from build123d import *

# Parameters (mm, degrees)
CORPS_D_PLACER_COPIER2_DEPTH = 104.8
BOSS_EXTRU_1_DEPTH           = 20
BOSS_EXTRU_1_DEPTH_BACK      = 130
ESQUISSE1_R                  = 5


with BuildPart() as part:
    # Corps-Déplacer/Copier2: read off the stored shape, not the designer's step
    # Corps-Déplacer/Copier2 outline → Corps-Déplacer/Copier2 (new body)
    with BuildSketch(Plane(origin=(0, 0, 0), x_dir=(1, 0, 0), z_dir=(0, 1, 0))):
        Polygon((7, 7), (-7, 7), (-7, -7), (7, -7), (11, 0), align=None)
    extrude(amount=CORPS_D_PLACER_COPIER2_DEPTH)

    # Corps-D_placer_Copier2 2 outline → Corps-D_placer_Copier2 2 (revolve, cut)
    with BuildSketch(Plane.XY):
        with BuildLine():
            Line((11, 104.8), (5, 104.8))
            ThreePointArc((5, 104.8), (8.003766504, 104.724764387), (11, 104.499246226))
            Line((11, 104.499246226), (11, 104.8))
        make_face()
    revolve(axis=Axis((0, 0, 0), (0, 1, 0)), mode=Mode.SUBTRACT)

    # Esquisse1 → Boss.-Extru.1 (add, two sides: drawn at the far end of the back side and taken through both)
    with BuildSketch(Plane.XZ.offset(-BOSS_EXTRU_1_DEPTH_BACK)):
        with Locations(Location((0, 0, 0), (0, 0, 270))):
            Circle(ESQUISSE1_R)
    extrude(amount=BOSS_EXTRU_1_DEPTH + BOSS_EXTRU_1_DEPTH_BACK)


solid = part.part
Work out the finished part from the listing and answer in its coordinate system (mm). A direction names the side the tool comes from. Round coordinates to 2 decimals unless told otherwise and drop trailing zeros. Write each loop counter-clockwise with the first axis right and the second up, starting at its lowest first coordinate (ties: lowest second). Pieces come first, ordered by that corner, then holes.
1) Given pin 1 Ø1.5 at (y, z) = (45, 3.5) entering from +X; pin 2 Ø3 at (y, z) = (64.5, -2) entering from +X; pin 3 Ø1 at (x, z) = (7.5, 0) entering from -Y, each flat-ended and moving along its own axis, determine where each tip first touches the part or whether it passes through.
2) The mould has two halves that part along Z. Classify faces 1 (the flat face through (0, -20, 0)), 2 (the cylindrical face through (-4.88, -9.86, 1.08)), 3 (the flat face through (0, 52, -7)), 4 (the flat face through (9, 51.6, 3.5)): pulls with the +Z half, pulls with the -Z half, needs draft (parallel to the pull), parting line crosses it, or undercut.
3) Straight lines are drawn through the part: line 1 (Y direction, x = 6.75, z = 3); line 2 (X direction, y = 80.5, z = 4.75); line 3 (Y direction, x = 8.5, z = -4.25). For each, find the intervals that lie inside material, in ascending order.
4) A tool of negligible diameter and unlimited length cuts with its end or side. For faces 5 (the cylindrical face through (1.5, 117.58, -4.77)), 6 (the flat face through (6, 0, 0)), 7 (the flat face through (0, 130, 0)), from which of +Z, -Z, +X, -X, +Y, -Y can it reach the whole face along a straight path? Write none if from no direction.
5) A cutting plane is placed at A-A (y = 100). Give the vertices of the cut face in (x, z).
Completed:
1. pin 1: stops at x = 9.43
1. pin 2: stops at x = 10.71
1. pin 3: stops at y = 0
2. face 1: needs draft
2. face 2: parting line crosses it
2. face 3: pulls with the -Z half
2. face 4: pulls with the +Z half
3. line 1: y = 0 to 104.75
3. line 2: x = -7 to 8.29
3. line 3: y = 0 to 104.63
4. face 5: +Y
4. face 6: -Y
4. face 7: +Z, -Z, +X, -X, +Y
5. outline: (-7, -7) - (7, -7) - (11, 0) - (7, 7) - (-7, 7) - close
